Autodesk Inventor part; units mm, degrees
ref_plane "YZ Plane" through (0, 0, 0) normal (1, 0, 0) x (0, 1, 0)
ref_plane "XZ Plane" through (0, 0, 0) normal (0, 1, 0) x (-1, 0, 0)
ref_plane "XY Plane" through (0, 0, 0) normal (0, 0, 1) x (1, 0, 0)
sketch "Sketch1" plane through (0, 0, 0) normal (0, 0, 1) x (1, 0, 0)
  arc A0 (-11.176, -9.652) -> (-9.652, -11.176) centre (-9.652, -9.652) ccw
  line L0 (-11.176, 9.652) -> (-11.176, -9.652)
  arc A1 (-9.652, 11.176) -> (-11.176, 9.652) centre (-9.652, 9.652) ccw
  line L1 (9.652, 11.176) -> (-9.652, 11.176)
  arc A2 (11.176, 9.652) -> (9.652, 11.176) centre (9.652, 9.652) ccw
  line L2 (11.176, -9.652) -> (11.176, 9.652)
  arc A3 (9.652, -11.176) -> (11.176, -9.652) centre (9.652, -9.652) ccw
  line L3 (-9.652, -11.176) -> (9.652, -11.176)
  arc A4 (12.7, 10.5918) -> (10.5918, 12.7) centre (10.5918, 10.5918) ccw
  line L4 (10.5918, 12.7) -> (-10.5918, 12.7)
  arc A5 (-10.5918, 12.7) -> (-12.7, 10.5918) centre (-10.5918, 10.5918) ccw
  line L5 (-12.7, 10.5918) -> (-12.7, 6.731)
  arc A6 (-13.081, 6.35) -> (-12.7, 6.731) centre (-13.081, 6.731) ccw
  line L6 (-13.081, 6.35) -> (-25.019, 6.35)
  arc A7 (-25.019, 6.35) -> (-25.4, 5.969) centre (-25.019, 5.969) ccw
  line L7 (-25.4, 5.969) -> (-25.4, 4.826)
  arc A8 (-25.4, 4.826) -> (-24.638, 4.064) centre (-24.638, 4.826) ccw
  line L8 (-24.638, 4.064) -> (-23.0632, 4.064)
  arc A9 (-23.0632, 4.064) -> (-22.6822, 4.445) centre (-23.0632, 4.445) ccw
  arc A10 (-22.3012, 4.826) -> (-22.6822, 4.445) centre (-22.3012, 4.445) ccw
  line L9 (-22.3012, 4.826) -> (-13.081, 4.826)
  arc A11 (-12.7, 4.445) -> (-13.081, 4.826) centre (-13.081, 4.445) ccw
  line L10 (-12.7, 4.445) -> (-12.7, -4.445)
  arc A12 (-13.081, -4.826) -> (-12.7, -4.445) centre (-13.081, -4.445) ccw
  line L11 (-13.081, -4.826) -> (-22.3012, -4.826)
  arc A13 (-22.6822, -4.445) -> (-22.3012, -4.826) centre (-22.3012, -4.445) ccw
  arc A14 (-22.6822, -4.445) -> (-23.0632, -4.064) centre (-23.0632, -4.445) ccw
  line L12 (-23.0632, -4.064) -> (-24.638, -4.064)
  arc A15 (-24.638, -4.064) -> (-25.4, -4.826) centre (-24.638, -4.826) ccw
  line L13 (-25.4, -4.826) -> (-25.4, -5.969)
  arc A16 (-25.4, -5.969) -> (-25.019, -6.35) centre (-25.019, -5.969) ccw
  line L14 (-25.019, -6.35) -> (-13.081, -6.35)
  arc A17 (-12.7, -6.731) -> (-13.081, -6.35) centre (-13.081, -6.731) ccw
  line L15 (-12.7, -6.731) -> (-12.7, -10.5918)
  arc A18 (-12.7, -10.5918) -> (-10.5918, -12.7) centre (-10.5918, -10.5918) ccw
  line L16 (-10.5918, -12.7) -> (10.5918, -12.7)
  arc A19 (10.5918, -12.7) -> (12.7, -10.5918) centre (10.5918, -10.5918) ccw
  line L17 (12.7, -10.5918) -> (12.7, 10.5918)
  point P0 (0, 0)
extrude "Extrusion1" add sketch "Sketch1" against normal blind 304.8
properties part number "9025"
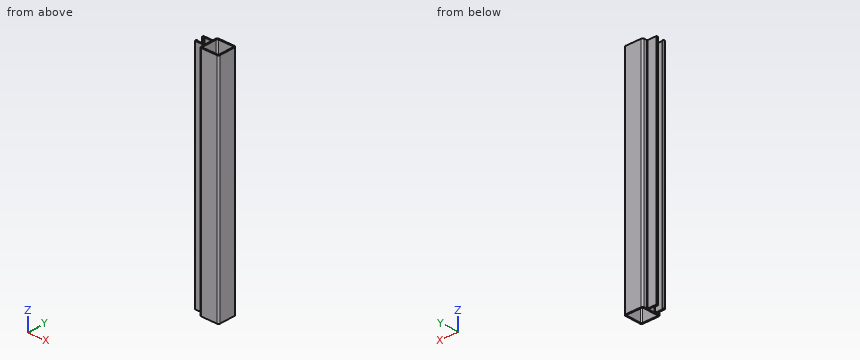
The listing builds one solid part. Answer for the finished solid, in the listing's coordinates (mm). Give positions to 0.01 mm unless a question says otherwise; leave off trailing zeros. Order: outer loops, then holes, each group sorted by start corner. A loop starts at its lowest first (then second) coordinate and runs counter-clockwise, first axis right, second up. Notation, with made-up numbers: M 9.25,-20.75 L 64.25,-20.75 A15 ccw 64.25,-8.75 Z; hole C 62.5,8 d1. An arc over 180 degrees is marked long. Put each result on its own line as item: value. Start each with the question number.
Item 1: The part is cut by section A-A, the plane x = -1. Determine the outline of the cut face in (y, z), and give its area (3 significant figures).
Item 2: Flat-ended cylindrical pins translate along their axes: P1, Ø9.5, axis at x = -19, z = -114, coming from the +Y side; P2, Ø1.2, axis at y = -8.5, z = -92, coming from the -X side; P3, Ø4, axis at y = 4.5, z = -157, coming from the -X side; P4, Ø10, axis at x = -18, z = -120, coming from the +Y side. Find the tip coordinate at first contact, or state that the pin passes through.
Item 3: Find the intervals of material crossed by line 1 along X through (y, z) = (7.75, -134); line 2 along X through (y, z) = (-10, -143), in increasing order.
Answer key:
1. outline: M -12.7,-304.8 L -11.18,-304.8 L -11.18,0 L -12.7,0 Z; M 11.18,-304.8 L 12.7,-304.8 L 12.7,0 L 11.18,0 Z
1. area: 929 mm²
2. P1: stops at y = 6.35
2. P2: stops at x = -12.7
2. P3: stops at x = -25.4
2. P4: stops at y = 6.36
3. line 1: x = -12.7 to -11.18, 11.18 to 12.7
3. line 2: x = -12.7 to -11.14, 11.14 to 12.7
